The model under review builds one solid part; all positions refer to its coordinate system, in mm. A direction names the side the tool comes from. Round coordinates to 2 decimals unless told otherwise and drop trailing zeros. Loops run counter-clockwise (first coordinate to the right, second up) from the corner with the lowest first, then second, coordinate; pieces in that order, holes last. Notation, with made-up numbers: M -27.75,6 L -3.75,6 A29 ccw -3.75,33 Z; hole C 25,31.25 d8. An arc over 180 degrees is marked long. Use a Markdown table: item, result. Add a question column.
```python
from build123d import *

# Parameters (mm, degrees)
SKETCH1_W                      = 177.8
SKETCH1_H                      = 203.2
BOSS_EXTRUDE1_DEPTH            = 76.2
F_6_0_204_DIAMETER_HOLE1_D     = 5.1816
F_6_0_204_DIAMETER_HOLE1_DEPTH = 11.938
F_6_0_204_DIAMETER_HOLE1_TIP   = 1.556709692
CUT_EXTRUDE1_START             = -50.8
CUT_EXTRUDE1_DEPTH             = 50.8


with BuildPart() as part:
    # Sketch1 → Boss-Extrude1 (new body)
    with BuildSketch(Plane(origin=(0, 0, 0), x_dir=(1, 0, 0), z_dir=(0, 1, 0))):
        Rectangle(SKETCH1_W, SKETCH1_H)
    extrude(amount=BOSS_EXTRUDE1_DEPTH)

    # #6 (0.204) Diameter Hole1
    with Locations(Plane(origin=(0, 76.2, 0), x_dir=(1, 0, 0), z_dir=(0, 1, 0))):
        with Locations((76.2, 88.9), (76.2, -88.9), (-76.2, -88.9), (-76.2, 88.9)):
            Hole(F_6_0_204_DIAMETER_HOLE1_D / 2, depth=F_6_0_204_DIAMETER_HOLE1_DEPTH)
            with Locations((0, 0, -(F_6_0_204_DIAMETER_HOLE1_DEPTH + F_6_0_204_DIAMETER_HOLE1_TIP / 2))):  # 118° drill point
                Cone(0, F_6_0_204_DIAMETER_HOLE1_D / 2, F_6_0_204_DIAMETER_HOLE1_TIP, mode=Mode.SUBTRACT)

    # Sketch4 → Cut-Extrude1 (cut)
    with BuildSketch(Plane(origin=(0, 76.2, 0), x_dir=(1, 0, 0), z_dir=(0, 1, 0)).offset(CUT_EXTRUDE1_START)):
        with BuildLine():
            ThreePointArc((-37.567106623, -6.35), (38.1, 0), (-37.567106623, 6.35))
            Line((-37.567106623, 6.35), (-88.9, 6.35))
            Line((-88.9, 6.35), (-88.9, -6.35))
            Line((-88.9, -6.35), (-37.567106623, -6.35))
        make_face()
    extrude(amount=CUT_EXTRUDE1_DEPTH, mode=Mode.SUBTRACT)


solid = part.part
```
(1) Consider section C-C, the plane x = -20.5. Give the boundary of the cut face in (y, z).
(2) To check wall thickness, follow probe 1 along Z at (x, y) = (76.2, 70); probe 2 along Z at (x, y) = (-76, 71); probe 3 along Z at (x, y) = (0, 62.5). State the ranges of each line that lie inside material, in increasing order.
(3) Consider section B-B, the plane z = 0. Give the boundary of the cut face in (x, y), then the cut area to 3 significant figures.
(4) Insertion check: pin 1 Ø4.5 at (x, z) = (76.2, 88.9) entering from -Y; pin 2 Ø23 at (x, z) = (-12, 17) entering from +Y. Each pin has a flat end and moves straight along its axis. Give the tip position at first contact, or say it passes through.
(5) For faces 1 (the face through (-88.9, 21, 1)), 2 (the face through (-64, 50, 6.35)), 3 (the face through (38.067, 50.444, 1.586)), list the 3-axis set-ups (+Z, -Z, +X, -X, +Y, -Y) from which the entire face can be reached by the end or side of a thin tool; tool diameter is ignored.
(6) Draft analysis for pull direction Z (two halves, no side actions). For faces 4 (the face through (74.807, 70.147, -91.085)), 5 (the face through (-1, 0, -1)), 6 (the face through (-1, 38, 101.6)), state which applies: released by +Z, released by -Z, zero draft, split by the parting line, or undercut.
(7) Consider section A-A, the plane y = 32.5. Give the boundary of the cut face in (x, z), then the cut area to 3 significant figures.
Found:
| question | item | result |
|---|---|---|
| 1 | outline | M 0,-101.6 L 76.2,-101.6 L 76.2,-32.11 L 25.4,-32.11 L 25.4,32.11 L 76.2,32.11 L 76.2,101.6 L 0,101.6 Z |
| 2 | probe 1 | z = -101.6 to -91.49, -86.31 to 86.31, 91.49 to 101.6 |
| 2 | probe 2 | z = -101.6 to -91.48, -86.32 to -6.35, 6.35 to 86.32, 91.48 to 101.6 |
| 2 | probe 3 | z = -101.6 to -38.1, 38.1 to 101.6 |
| 3 | outline | M -88.9,0 L 88.9,0 L 88.9,76.2 L 38.1,76.2 L 38.1,25.4 L -88.9,25.4 Z |
| 3 | area | 7,100 mm^2 |
| 4 | pin 1 | stops at y = 0 |
| 4 | pin 2 | stops at y = 25.4 |
| 5 | face 1 | +Z, -Z, -X, +Y, -Y |
| 5 | face 2 | -X, +Y |
| 5 | face 3 | +Y |
| 6 | face 4 | undercut |
| 6 | face 5 | zero draft |
| 6 | face 6 | released by +Z |
| 7 | outline | M -88.9,-101.6 L 88.9,-101.6 L 88.9,101.6 L -88.9,101.6 L -88.9,6.35 L -37.57,6.35 A38.1 cw long -37.57,-6.35 L -88.9,-6.35 Z |
| 7 | area | 30,900 mm^2 |
